Autodesk Inventor part; units mm, degrees
ref_plane "YZ Plane" through (0, 0, 0) normal (1, 0, 0) x (0, 1, 0)
ref_plane "XZ Plane" through (0, 0, 0) normal (0, 1, 0) x (-1, 0, 0)
ref_plane "XY Plane" through (0, 0, 0) normal (0, 0, 1) x (1, 0, 0)
sketch "Sketch2" plane through (0, 0, 0) normal (0, 0, 1) x (1, 0, 0)
  line L0 (0, 0) -> (-101.6, 0)
  line L1 (-101.6, 0) -> (-101.6, 101.6)
  line L2 (-101.6, 101.6) -> (0, 101.6)
  line L3 (0, 101.6) -> (0, 0)
  circle A0 centre (-12.7, 88.9) radius 2.5797
  circle A1 centre (-50.8, 76.2) radius 9.525
  circle A2 centre (-25.4, 38.1) radius 2.5797
  circle A3 centre (-50.8, 25.4) radius 9.525
  circle A4 centre (-88.9, 88.9) radius 2.5797
  circle A5 centre (-12.7, 63.5) radius 2.5797
  circle A6 centre (-88.9, 63.5) radius 2.5797
  circle A7 centre (-76.2, 38.1) radius 2.5797
  circle A8 centre (-25.4, 12.7) radius 2.5797
  circle A9 centre (-76.2, 12.7) radius 2.5797
  line L4 (-85.725, 19.05) -> (-101.6, 19.05)
  line L5 (-101.6, 19.05) -> (-101.6, 22.225)
  line L6 (-101.6, 22.225) -> (-85.725, 22.225)
  line L7 (-85.725, 22.225) -> (-85.725, 19.05)
  line L8 (-101.6, 22.225) -> (-85.725, 22.225)
  line L9 (-85.725, 22.225) -> (-85.725, 23.8125)
  line L10 (-85.725, 23.8125) -> (-101.6, 23.8125)
  line L11 (-101.6, 23.8125) -> (-101.6, 22.225)
  line L12 (-85.725, 23.8125) -> (-101.6, 23.8125)
  line L13 (-101.6, 23.8125) -> (-101.6, 26.9875)
  line L14 (-101.6, 26.9875) -> (-85.725, 26.9875)
  line L15 (-85.725, 26.9875) -> (-85.725, 23.8125)
  line L16 (-101.6, 26.9875) -> (-85.725, 26.9875)
  line L17 (-85.725, 26.9875) -> (-85.725, 28.575)
  line L18 (-85.725, 28.575) -> (-101.6, 28.575)
  line L19 (-101.6, 28.575) -> (-101.6, 26.9875)
  line L20 (-85.725, 28.575) -> (-101.6, 28.575)
  line L21 (-101.6, 28.575) -> (-101.6, 31.75)
  line L22 (-101.6, 31.75) -> (-85.725, 31.75)
  line L23 (-85.725, 31.75) -> (-85.725, 28.575)
  line L24 (-85.725, 31.8135) -> (-101.6, 31.8135)
  line L25 (-101.6, 31.8135) -> (-101.6, 28.5115)
  line L26 (-101.6, 28.5115) -> (-85.725, 28.5115)
  line L27 (-85.725, 28.5115) -> (-85.725, 31.8135)
  line L28 (-85.725, 27.051) -> (-101.6, 27.051)
  line L29 (-101.6, 27.051) -> (-101.6, 23.749)
  line L30 (-101.6, 23.749) -> (-85.725, 23.749)
  line L31 (-85.725, 23.749) -> (-85.725, 27.051)
  line L32 (-85.725, 22.2885) -> (-101.6, 22.2885)
  line L33 (-101.6, 22.2885) -> (-101.6, 18.9865)
  line L34 (-101.6, 18.9865) -> (-85.725, 18.9865)
  line L35 (-85.725, 18.9865) -> (-85.725, 22.2885)
  line L36 (-101.6, 26.4583) -> (-85.725, 26.4583)
  line L37 (-85.725, 26.4583) -> (-85.725, 24.3417)
  line L38 (-85.725, 24.3417) -> (-101.6, 24.3417)
  line L39 (-101.6, 24.3417) -> (-101.6, 26.4583)
  line L40 (-50.8, 0) -> (-50.8, 101.6)
  line L41 (-15.875, 19.05) -> (0, 19.05)
  line L42 (0, 19.05) -> (0, 22.225)
  line L43 (0, 22.225) -> (-15.875, 22.225)
  line L44 (-15.875, 22.225) -> (-15.875, 19.05)
  line L45 (0, 22.225) -> (-15.875, 22.225)
  line L46 (-15.875, 22.225) -> (-15.875, 23.8125)
  line L47 (-15.875, 23.8125) -> (0, 23.8125)
  line L48 (0, 23.8125) -> (0, 22.225)
  line L49 (-15.875, 23.8125) -> (0, 23.8125)
  line L50 (0, 23.8125) -> (0, 26.9875)
  line L51 (0, 26.9875) -> (-15.875, 26.9875)
  line L52 (-15.875, 26.9875) -> (-15.875, 23.8125)
  line L53 (0, 26.9875) -> (-15.875, 26.9875)
  line L54 (-15.875, 26.9875) -> (-15.875, 28.575)
  line L55 (-15.875, 28.575) -> (0, 28.575)
  line L56 (0, 28.575) -> (0, 26.9875)
  line L57 (-15.875, 28.575) -> (0, 28.575)
  line L58 (0, 28.575) -> (0, 31.75)
  line L59 (0, 31.75) -> (-15.875, 31.75)
  line L60 (-15.875, 31.75) -> (-15.875, 28.575)
  line L61 (-15.875, 31.8135) -> (0, 31.8135)
  line L62 (0, 31.8135) -> (0, 28.5115)
  line L63 (0, 28.5115) -> (-15.875, 28.5115)
  line L64 (-15.875, 28.5115) -> (-15.875, 31.8135)
  line L65 (-15.875, 27.051) -> (0, 27.051)
  line L66 (0, 27.051) -> (0, 23.749)
  line L67 (0, 23.749) -> (-15.875, 23.749)
  line L68 (-15.875, 23.749) -> (-15.875, 27.051)
  line L69 (-15.875, 22.2885) -> (0, 22.2885)
  line L70 (0, 22.2885) -> (0, 18.9865)
  line L71 (0, 18.9865) -> (-15.875, 18.9865)
  line L72 (-15.875, 18.9865) -> (-15.875, 22.2885)
  line L73 (0, 26.4583) -> (-15.875, 26.4583)
  line L74 (-15.875, 26.4583) -> (-15.875, 24.3417)
  line L75 (-15.875, 24.3417) -> (0, 24.3417)
  line L76 (0, 24.3417) -> (0, 26.4583)
  point P0 (-101.6, 30.1625)
  point P1 (-101.6, 20.6375)
  point P2 (-101.6, 25.4)
  point P3 (-85.725, 25.4)
  point P4 (0, 30.1625)
  point P5 (0, 20.6375)
  point P6 (0, 25.4)
  point P7 (-15.875, 25.4)
  point P8 (-50.8, 15.875)
  point P9 (-50.8, 34.925)
  point P10 (-50.8, 66.675)
  point P11 (-50.8, 85.725)
  dimension "d60" = 101.6
  dimension "d61" = 101.6
  dimension "d62" = 19.05
  dimension "d63" = 5.1594
  dimension "d66" = 12.7
  dimension "d69" = 76.2
  dimension "d72" = 25.4
  dimension "d75" = 12.7
  dimension "d76" = 38.1
  dimension "d77" = 12.7
  dimension "d80" = 50.8
  dimension "d83" = 25.4
  dimension "d86" = 25.4
  dimension "d87" = 12.7
  dimension "d88" = 12.7
  dimension "d89" = 25.4
  dimension "d96" = 3.175
  dimension "d97" = 1.5875
  dimension "d98" = 3.302
  dimension "d101" = 2.1167
  dimension "d103" = 15.875
  dimension "d104" = 25.4
extrude "Extrusion2" add sketch "Sketch2" along normal blind 3.175 contours L0 L40 A3 A1 L2 L3 L61 L64 L60 L54 L52 L46 L44 L72 L71 | L0 L1 L34 L35 L7 L9 L15 L17 L23 L27 L24 L2 L40 A1 A3 | L40 A1 | A1 L40 | L69 L46 L67 L3 | L67 L46 L47 L3 | L1 L30 L9 L32 | L47 L52 L75 L3 | L1 L10 L9 L30 | L75 L52 L73 L3 | L1 L38 L15 L10 | L73 L52 L51 L3 | L1 L36 L15 L38 | L51 L54 L65 L3 | L1 L14 L15 L36 | L65 L54 L63 L3 | L1 L28 L17 L14 | L26 L17 L28 L1
fillet "Fillet3" radius 3.175 8 edges at (0, 101.6, 1.5875) (-101.6, 101.6, 1.5875) (0, 18.9865, 1.5875) (0, 31.8135, 1.5875) (0, 0, 1.5875) (-101.6, 0, 1.5875) (-101.6, 18.9865, 1.5875) (-101.6, 31.8135, 1.5875)
fillet "Fillet4" radius 1.5875 4 edges at (0, 22.2885, 1.5875) (0, 28.5115, 1.5875) (-101.6, 22.2885, 1.5875) (-101.6, 28.5115, 1.5875)
properties part number "Dipper Plate (backplate)"
Can you work these out from the model? Positions are in its coordinate system, mm. A direction names the side the tool comes from. Coordinates: 2 decimals unless noted, no trailing zeros. Loops run counter-clockwise (first coordinate to the right, second up) from the corner with the lowest first, then second, coordinate; pieces in that order, holes last. Notation, with made-up numbers: (-2.5, 17) - (16.5, 17) arc R18 cw to (16.5, 46) - close; hole circle Ø11 at (30.25, -38). An arc over 180 degrees is marked (long way). Put each result on its own line as item: value. Start each with the question number.
Item 1: If I drill on line 1 along Y through (x, z) = (-76.2, 2.4); line 2 along Y through (x, z) = (-92, 0.9); line 3 along Y through (x, z) = (-88.9, 1), over which ranges is the centre line in solid material (lowest first)?
Item 2: For pin 1 (8.5 mm diameter, centred on x = -25.4, y = 12.7, fed in from +Z) (3 decimals); pin 2 (1 mm diameter, centred on y = 21, z = 1, fed in from +X) (3 decimals); pin 3 (1.6 mm diameter, centred on y = 20.5, z = 1, fed in from -X) (3 decimals), each with a flat end and sliding along its axis, tell me the tip position at first contact or that it passes through.
Item 3: Suppose I cut it at C-C (x = -12.7). Please give me the cut outline in (y, z) (1 decimal), and give its area (3 significant figures).
Item 4: Suppose I cut it at A-A (y = 63.5). Please give me the cut outline in (x, z) (3 decimals), and give its area (3 significant figures).
Item 5: If we mould it in two halves opening along X, with no side actions, what happens to faces 1 (the face through (-27.977, 12.587, 1.565)), 2 (the face through (-52, 52, 0)), 3 (the face through (-0.955, 32.719, 1.61))? For each: +X half, -X half, draft (parallel to the pull), parting line (faces both ways), or undercut.
Item 6: Which directions (+Z, -Z, +X, -X, +Y, -Y) give clear straight access to the entire face, cutting with the end or side of a thin tool? Please do faces 4 (the face through (-10, 31.814, 2)), 5 (the face through (-92, 31.814, 2)), 6 (the face through (0, 67, 2)).
Item 7: Suppose I cut it at B-B (x = -25.4). Please give me the cut outline in (y, z) (3 decimals), and give its area (3 significant figures).
Item 8: Suppose I cut it at D-D (z = 1.65). State how many separate pieces and enclosed holes the cut face has, and give its area (3 significant figures).
Here are the results:
1. line 1: 0 to 10.12, 15.28 to 35.52, 40.68 to 101.6
1. line 2: 0 to 18.99, 22.29 to 28.51, 31.81 to 101.6
1. line 3: 0 to 18.99, 22.29 to 28.51, 31.81 to 60.92, 66.08 to 86.32, 91.48 to 101.6
2. pin 1: z = 3.175
2. pin 2: x = -15.875
2. pin 3: x = -85.725
3. outline: (0, 0) - (19, 0) - (19, 3.2) - (0, 3.2) - close; (22.3, 0) - (28.5, 0) - (28.5, 3.2) - (22.3, 3.2) - close; (31.8, 0) - (60.9, 0) - (60.9, 3.2) - (31.8, 3.2) - close; (66.1, 0) - (86.3, 0) - (86.3, 3.2) - (66.1, 3.2) - close; (91.5, 0) - (101.6, 0) - (101.6, 3.2) - (91.5, 3.2) - close
3. area: 269 mm²
4. outline: (-101.6, 0) - (-91.48, 0) - (-91.48, 3.175) - (-101.6, 3.175) - close; (-86.32, 0) - (-15.28, 0) - (-15.28, 3.175) - (-86.32, 3.175) - close; (-10.12, 0) - (0, 0) - (0, 3.175) - (-10.12, 3.175) - close
4. area: 290 mm²
5. face 1: undercut
5. face 2: draft
5. face 3: +X half
6. face 4: +Z, -Z, +X
6. face 5: +Z, -Z, -X
6. face 6: +Z, -Z, +X, +Y, -Y
7. outline: (0, 0) - (10.12, 0) - (10.12, 3.175) - (0, 3.175) - close; (15.28, 0) - (35.52, 0) - (35.52, 3.175) - (15.28, 3.175) - close; (40.68, 0) - (101.6, 0) - (101.6, 3.175) - (40.68, 3.175) - close
7. area: 290 mm²
8. separate pieces: 1
8. enclosed holes: 9
8. area: 9,640 mm²
